Could you check a few things on this drawing? It's one solid part, dimensions in mm from its lowest x, y, z. A direction names the side the tool comes from. Round coordinates to 2 decimals unless told otherwise and drop trailing zeros. Write each loop counter-clockwise with the first axis right and the second up, starting at its lowest first coordinate (ties: lowest second). Pieces come first, ordered by that corner, then holes. Notation, with made-up numbers: (35.25, 40) -> (48.25, 40) arc R29 ccw to (48.25, 74) -> close; hole circle Ø4 at (39, 43). An arc over 180 degrees is marked (long way). Put each result on its own line as item: value. Start each with the question number.
1) Will these pins go through, and if not, where does the flat tip stop? P1, Ø1, axis at x = 11, y = 17.5, coming from the +Z side; P2, Ø1, axis at y = 15.5, z = 16.5, coming from the -X side; P3, Ø1.5, axis at x = 3, y = 3, coming from the +Z side.
2) Which directions (+Z, -Z, +X, -X, +Y, -Y) give clear straight access to the entire face, cutting with the end or side of a thin tool? Please do the marked faces 4 and 5.
3) I want a section at D-D, the plane z = 17.5. List the corners of the cut face in (x, y) for me.
4) I want a section at B-B, the plane x = 7. List the corners of the cut face in (y, z) for me.
5) If I drill on line 1 along Z through (x, y) = (9.5, 15); line 2 along Z through (x, y) = (7.25, 3) (1 decimal), over which ranges is the centre line in solid material (lowest first)? Write a range as [from, to].
6) We'd pull the mould along X, two halves only. Please class the marked faces 1, 2 and 3: released by +X, released by -X, zero draft, split by the parting line, or undercut.
7) I want a section at A-A, the plane z = 12.25. List the corners of the cut face in (x, y) for me, then the cut area to 3 significant figures.
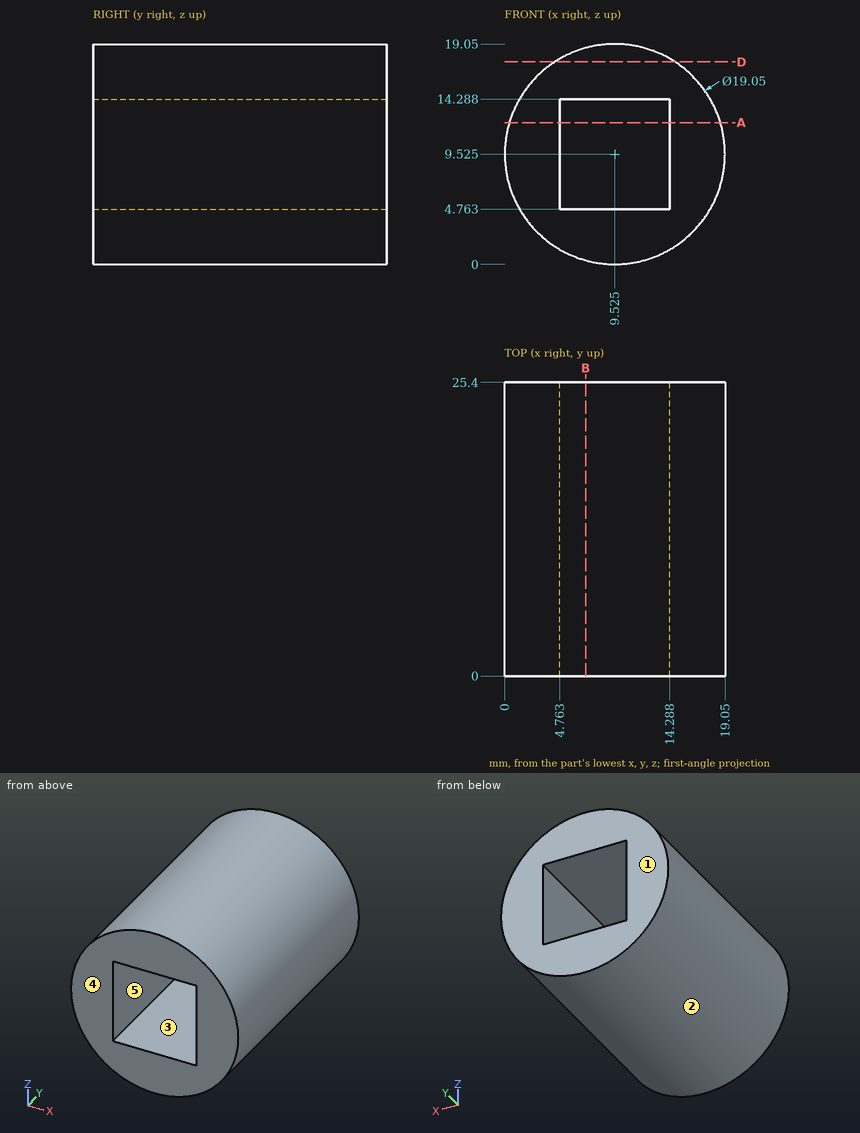
Findings:
1. P1: stops at z = 19
1. P2: stops at x = 2.54
1. P3: stops at z = 17.1
2. face 4: +Z, -Z, +X, -X, -Y
2. face 5: +Y, -Y
3. outline: (4.32, 0) -> (14.73, 0) -> (14.73, 25.4) -> (4.32, 25.4) -> close
4. outline: (0, 0.34) -> (25.4, 0.34) -> (25.4, 4.76) -> (0, 4.76) -> close; (0, 14.29) -> (25.4, 14.29) -> (25.4, 18.71) -> (0, 18.71) -> close
5. line 1: z = [0, 4.76], [14.29, 19.05]
5. line 2: z = [0.3, 4.8], [14.3, 18.8]
6. face 1: zero draft
6. face 2: split by the parting line
6. face 3: undercut
7. outline: (0.4, 0) -> (4.76, 0) -> (4.76, 25.4) -> (0.4, 25.4) -> close; (14.29, 0) -> (18.65, 0) -> (18.65, 25.4) -> (14.29, 25.4) -> close
7. area: 222 mm2
